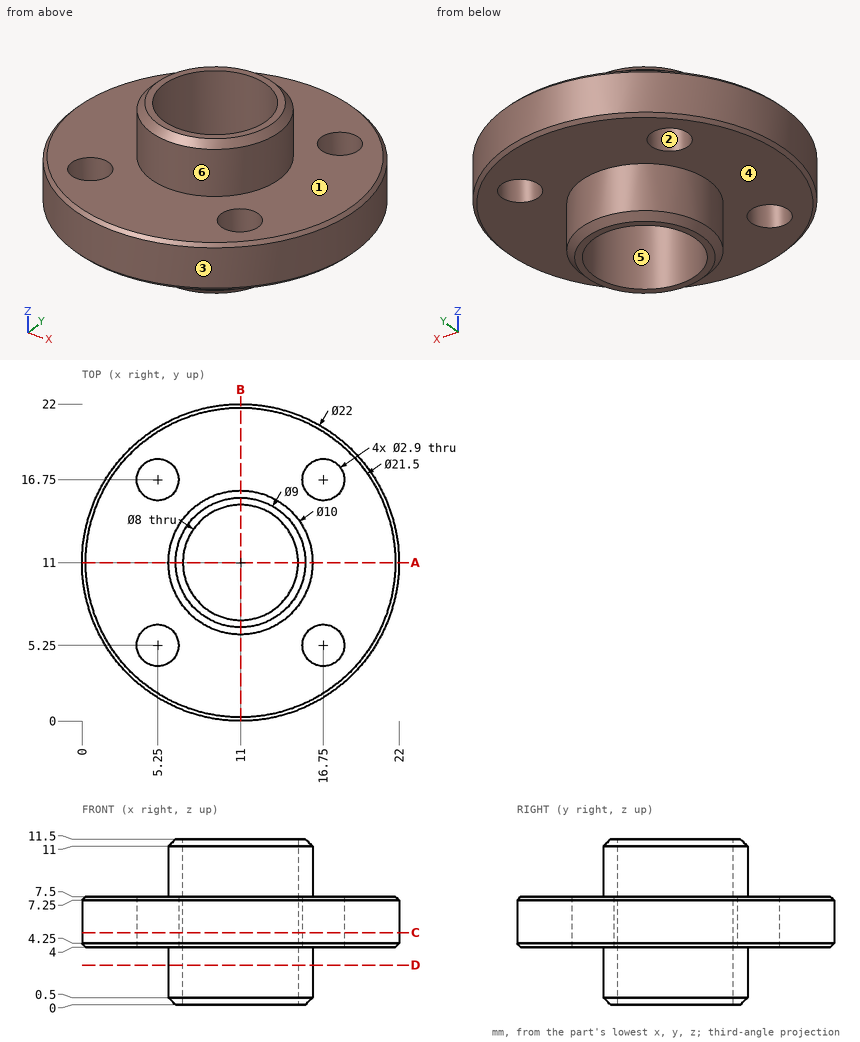
For this review, use the dimensioned drawing (mm, ordinates from the lowest corner) and the shaded views. A direction names the side the tool comes from. Round coordinates to 2 decimals unless told otherwise and drop trailing zeros. Order: outer loops, then holes, each group sorted by start corner. A loop starts at its lowest first (then second) coordinate and runs counter-clockwise, first axis right, second up. Notation, with made-up numbers: (34, 87.5) - (56, 87.5) arc R14 ccw to (56, 104.5) - close; hole circle Ø3 at (62, -11). An arc over 180 degrees is marked (long way). Use one line per item in the form item = value.
Q1. Add section C-C on z = 5. Give the boundary of the cut face in (x, y), then the cut area to 3 significant figures.
Response values:
outline = circle Ø22 at (11, 11); hole circle Ø2.9 at (5.25, 5.25); hole circle Ø2.9 at (5.25, 16.75); hole circle Ø8 at (11, 11); hole circle Ø2.9 at (16.75, 5.25); hole circle Ø2.9 at (16.75, 16.75)
area = 303 mm^2
Q2. To check wall thickness, follow line 1 (Y direction, x = 5.25, z = 5.7); line 2 (Y direction, x = 4.75, z = 6); line 3 (X direction, y = 10.75, z = 1.5). State the ranges of each line that lie inside material, in increasing order.
Response values:
line_1 = 1.62 to 3.8, 6.7 to 15.3, 18.2 to 20.38
line_2 = 1.95 to 3.89, 6.61 to 15.39, 18.11 to 20.05
line_3 = 6.01 to 7.01, 14.99 to 15.99
Q3. Add section D-D on z = 2.75. Give the boundary of the cut face in (x, y), then the cut area to 3 significant figures.
Response values:
outline = circle Ø10 at (11, 11); hole circle Ø8 at (11, 11)
area = 28.3 mm^2
Q4. Mouldability with a two-part tool opening along Y and no side actions: class the marked faces 1, 2 and 3 as pulls with the +Y half, pulls with the -Y half, needs draft (parallel to the pull), parting line crosses it, or undercut.
Response values:
face_1 = needs draft
face_2 = undercut
face_3 = parting line crosses it
Q5. Clearance check with flat-ended pins moving along their axes: P1, Ø1, axis at y = 17.5, z = 4.5, coming from the +X side; P2, Ø5, axis at y = 17.5, z = 3, coming from the -X side; P3, Ø4.5, axis at x = 5.25, y = 16.75, coming from the +Z side. State where each tip first meets the part, or that it passes through.
Response values:
P1 = 20.22
P2 = 0.89
P3 = 7.5
Q6. Tool access review of the marked faces 4, 5 and 6: name each direction out of +Z, -Z, +X, -X, +Y, -Y from which nothing blocks a thin tool from reaching the whole face with its end or side.
Response values:
face_4 = -Z
face_5 = +Z, -Z
face_6 = +Z
Q7. Add section A-A on y = 11. Give the boundary of the cut face in (x, z).
Response values:
outline = (0, 4.25) - (0.25, 4) - (6, 4) - (6, 0.5) - (6.5, 0) - (7, 0) - (7, 11.5) - (6.5, 11.5) - (6, 11) - (6, 7.5) - (0.25, 7.5) - (0, 7.25) - close; (15, 0) - (15.5, 0) - (16, 0.5) - (16, 4) - (21.75, 4) - (22, 4.25) - (22, 7.25) - (21.75, 7.5) - (16, 7.5) - (16, 11) - (15.5, 11.5) - (15, 11.5) - close
